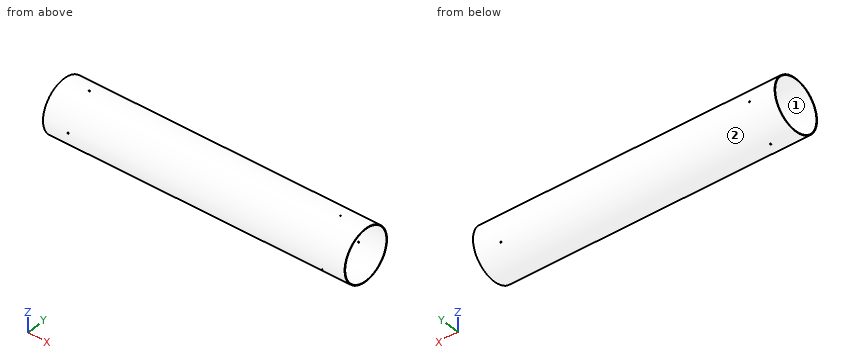
from build123d import *

# Parameters (mm, degrees)
SKETCH3_R               = 78.359
SKETCH3_R_2             = 76.2
BOSS_EXTRUDE1_DEPTH     = 914.4
CUT_EXTRUDE1_REACH      = 923.09
CUT_EXTRUDE1_END_RADIUS = 78.359
SKETCH4_R               = 1.41224
CIRPATTERN1_COUNT       = 3
CUT_EXTRUDE2_REACH      = 923.09
CUT_EXTRUDE2_END_RADIUS = 78.359
SKETCH5_R               = 1.7859375
CIRPATTERN2_COUNT       = 4


with BuildPart() as part:
    # Sketch3 → Boss-Extrude1 (new body)
    with BuildSketch(Plane(origin=(0, 0, 0), x_dir=(0, 0, -1), z_dir=(1, 0, 0))):
        Circle(SKETCH3_R)
        Circle(SKETCH3_R_2, mode=Mode.SUBTRACT)
    extrude(amount=BOSS_EXTRUDE1_DEPTH)

    # Cut-Extrude1: up to this cylinder (the profile starts inside it)
    cut_extrude1_end = Plane(origin=(838.2, 0, 0), z_dir=(-1, 0, 0)) * Cylinder(CUT_EXTRUDE1_END_RADIUS, 2003.898, mode=Mode.PRIVATE)
    # Sketch4 → Cut-Extrude1 (cut, up to the surface)
    with BuildSketch(Plane.XY, mode=Mode.PRIVATE) as cut_extrude1_sk1:
        with Locations(Location((838.2, 0, 0), (0, 0, 180))):
            Circle(SKETCH4_R)
    cut_extrude1_tool1 = extrude(cut_extrude1_sk1.sketch, amount=CUT_EXTRUDE1_REACH, mode=Mode.PRIVATE) & cut_extrude1_end
    cut_extrude1 = cut_extrude1_tool1.solids().sort_by_distance((838.2, 0, 0))[0]
    add(cut_extrude1, mode=Mode.SUBTRACT)

    # CirPattern1: Cut-Extrude1 ×3 about axis
    cirpattern1_axis = Axis((914.4, 0, 0), (1, 0, 0))
    for i in range(1, CIRPATTERN1_COUNT):
        add(cut_extrude1.rotate(cirpattern1_axis, i * 360 / CIRPATTERN1_COUNT), mode=Mode.SUBTRACT)

    # Cut-Extrude2: up to this cylinder (the profile starts inside it)
    cut_extrude2_end = Plane(origin=(76.2, 0, 0), z_dir=(-1, 0, 0)) * Cylinder(CUT_EXTRUDE2_END_RADIUS, 2003.898, mode=Mode.PRIVATE)
    # Sketch5 → Cut-Extrude2 (cut, up to the surface)
    with BuildSketch(Plane.XY, mode=Mode.PRIVATE) as cut_extrude2_sk1:
        with Locations(Location((76.2, 0, 0), (0, 0, 180))):
            Circle(SKETCH5_R)
    cut_extrude2_tool1 = extrude(cut_extrude2_sk1.sketch, amount=CUT_EXTRUDE2_REACH, mode=Mode.PRIVATE) & cut_extrude2_end
    cut_extrude2 = cut_extrude2_tool1.solids().sort_by_distance((76.2, 0, 0))[0]
    add(cut_extrude2, mode=Mode.SUBTRACT)

    # CirPattern2: Cut-Extrude2 ×4 about axis
    cirpattern2_axis = Axis((0, 0, 0), (1, 0, 0))
    for i in range(1, CIRPATTERN2_COUNT):
        add(cut_extrude2.rotate(cirpattern2_axis, i * 360 / CIRPATTERN2_COUNT), mode=Mode.SUBTRACT)


solid = part.part
Could you check a few things on this model? Use its own coordinates, in mm. Face numbers are marked on the shaded views. Round coordinates to 2 decimals unless told otherwise and drop trailing zeros. Write each loop counter-clockwise with the first axis right and the second up, starting at its lowest first coordinate (ties: lowest second). Pieces come first, ordered by that corner, then holes. Notation, with made-up numbers: (47.5, 7) - (61.5, 7) arc R14 cw to (61.5, 31) - close; hole circle Ø1 at (70.5, 86.25). An arc over 180 degrees is marked (long way). Put each result on its own line as item: value. Start each with the question number.
(1) I want a section at C-C, the plane x = 574.5. Please give me the cut outline in (y, z).
(2) I want a section at B-B, the plane y = -57.5. Please give me the cut outline in (x, z), plus the area to 3 significant figures.
(3) I need wall thicknesses on probe 1 along X at (y, z) = (77.75, 0); probe 2 along Y at (x, z) = (612.5, -0.5); probe 3 along Z at (x, y) = (120, -6). Which ranges of each line are inside material? Lowest first, please.
(4) Thinking about a two-plate mould opening in Z: for the marked faces 1 and 2, which applies, released by +Z, released by -Z, zero draft, split by the parting line, or undercut?
(5) I want a section at A-A, the plane z = -28.5. Please give me the cut outline in (x, y).
(6) Will these pins go through, and if not, where does the flat tip stop? pin 1 (2 mm diameter, centred on x = 76.2, z = 0, fed in from +Y); pin 2 (10 mm diameter, centred on x = 236, z = 36.5, fed in from +Y); pin 3 (5 mm diameter, centred on x = 111.5, z = -27.5, fed in from -Y); pin 4 (3 mm diameter, centred on x = 248, z = 41.5, fed in from -Y).
Here are the results:
1. outline: circle Ø156.72 at (0, 0); hole circle Ø152.4 at (0, 0)
2. outline: (0, -53.23) - (914.4, -53.23) - (914.4, -50) - (0, -50) - close; (0, 50) - (914.4, 50) - (914.4, 53.23) - (0, 53.23) - close
2. area: 5,910 mm^2
3. probe 1: x = 0 to 74.41, 77.99 to 914.4
3. probe 2: y = -78.36 to -76.2, 76.2 to 78.36
3. probe 3: z = -78.13 to -75.96, 75.96 to 78.13
4. face 1: undercut
4. face 2: split by the parting line
5. outline: (0, -72.99) - (914.4, -72.99) - (914.4, -70.67) - (0, -70.67) - close; (0, 70.67) - (914.4, 70.67) - (914.4, 72.99) - (0, 72.99) - close
6. pin 1: passes through
6. pin 2: stops at y = 71.75
6. pin 3: stops at y = -74.26
6. pin 4: stops at y = -67.38
